Read the model definition and answer for the solid it produces. Units are mm, in the model's axes. A direction names the side the tool comes from. Round coordinates to 2 decimals unless told otherwise and drop trailing zeros. Order: outer loops, then holes, each group sorted by start corner. A loop starts at its lowest first (then second) coordinate and runs counter-clockwise, first axis right, second up.
from build123d import *

# Parameters (mm, degrees)
SKETCH_W        = 200
SKETCH_H        = 90
SKETCH_R        = 1.5625
SKETCH_W_2      = 60
SKETCH_H_2      = 67
PAD_DEPTH       = 5
SKETCH002_W     = 41
SKETCH002_H     = 9.5
POCKET_DEPTH    = 5.001
SKETCH003_R     = 1.5625
POCKET001_DEPTH = 5.001
FILLET_R        = 30
FILLET001_R     = 4
FILLET002_R     = 4
FILLET003_R     = 4


with BuildPart() as part:
    # Sketch → Pad (new body)
    with BuildSketch(Plane.XY):
        with Locations((100, -45)):
            Rectangle(SKETCH_W, SKETCH_H)
        with Locations((185, -30)):
            Circle(SKETCH_R, mode=Mode.SUBTRACT)
        with Locations((185, -10)):
            Circle(SKETCH_R, mode=Mode.SUBTRACT)
        with Locations((175, -20)):
            Circle(SKETCH_R, mode=Mode.SUBTRACT)
        with Locations((175, -40)):
            Circle(SKETCH_R, mode=Mode.SUBTRACT)
        with Locations((25, -40)):
            Circle(SKETCH_R, mode=Mode.SUBTRACT)
        with Locations((25, -20)):
            Circle(SKETCH_R, mode=Mode.SUBTRACT)
        with Locations((15, -30)):
            Circle(SKETCH_R, mode=Mode.SUBTRACT)
        with Locations((15, -10)):
            Circle(SKETCH_R, mode=Mode.SUBTRACT)
        with Locations((70, -38.5)):
            Rectangle(SKETCH_W_2, SKETCH_H_2, mode=Mode.SUBTRACT)
        with BuildLine():
            ThreePointArc((158.0113, -7.9887), (155.0113, -4.9887), (152.0113, -7.9887))
            Line((152.0113, -7.9887), (152.0113, -17.9887))
            ThreePointArc((152.0113, -17.9887), (155.0113, -20.9887), (158.0113, -17.9887))
            Line((158.0113, -7.9887), (158.0113, -17.9887))
        make_face(mode=Mode.SUBTRACT)
        with BuildLine():
            ThreePointArc((151, -31.5), (131.5, -12), (112, -31.5))
            Line((112, -31.5), (112, -41.5))
            ThreePointArc((112, -41.5), (131.5, -61), (151, -41.5))
            Line((151, -31.5), (151, -41.5))
        make_face(mode=Mode.SUBTRACT)
        with BuildLine():
            ThreePointArc((158.0113, -55.0113), (155.0113, -52.0113), (152.0113, -55.0113))
            Line((152.0113, -55.0113), (152.0113, -65.0113))
            ThreePointArc((152.0113, -65.0113), (155.0113, -68.0113), (158.0113, -65.0113))
            Line((158.0113, -55.0113), (158.0113, -65.0113))
        make_face(mode=Mode.SUBTRACT)
        with BuildLine():
            ThreePointArc((110.9887, -55.0113), (107.9887, -52.0113), (104.9887, -55.0113))
            Line((104.9887, -55.0113), (104.9887, -65.0113))
            ThreePointArc((104.9887, -65.0113), (107.9887, -68.0113), (110.9887, -65.0113))
            Line((110.9887, -55.0113), (110.9887, -65.0113))
        make_face(mode=Mode.SUBTRACT)
        with BuildLine():
            ThreePointArc((110.9887, -7.9887), (107.9887, -4.9887), (104.9887, -7.9887))
            Line((104.9887, -7.9887), (104.9887, -17.9887))
            ThreePointArc((104.9887, -17.9887), (107.9887, -20.9887), (110.9887, -17.9887))
            Line((110.9887, -7.9887), (110.9887, -17.9887))
        make_face(mode=Mode.SUBTRACT)
    extrude(amount=PAD_DEPTH)

    # Sketch002 → Pocket (cut, through all)
    with BuildSketch(Plane.XY.offset(5)):
        with Locations((70, -76.75)):
            Rectangle(SKETCH002_W, SKETCH002_H)
    extrude(amount=-POCKET_DEPTH, mode=Mode.SUBTRACT)

    # Sketch003 → Pocket001 (cut, through all)
    with BuildSketch(Plane.XY.offset(5)):
        with Locations((25, -10)):
            Circle(SKETCH003_R)
        with Locations((15, -20)):
            Circle(SKETCH003_R)
        with Locations((15, -40)):
            Circle(SKETCH003_R)
        with Locations((25, -30)):
            Circle(SKETCH003_R)
        with Locations((175, -10)):
            Circle(SKETCH003_R)
        with Locations((185, -20)):
            Circle(SKETCH003_R)
        with Locations((185, -40)):
            Circle(SKETCH003_R)
        with Locations((175, -30)):
            Circle(SKETCH003_R)
    extrude(amount=-POCKET001_DEPTH, mode=Mode.SUBTRACT)

    # Fillet
    fillet_edges = [part.edges().sort_by_distance(p)[0] for p in [
        (200, -90, 2.5),
        (0, -90, 2.5),
    ]]
    fillet(fillet_edges, radius=FILLET_R)

    # Fillet001
    fillet001_edges = [part.edges().sort_by_distance(p)[0] for p in [
        (40, -72, 2.5),
        (49.5, -81.5, 2.5),
        (49.5, -72, 2.5),
        (100, -72, 2.5),
        (90.5, -72, 2.5),
        (90.5, -81.5, 2.5),
    ]]
    fillet(fillet001_edges, radius=FILLET001_R)

    # Fillet002
    fillet002_edges = [part.edges().sort_by_distance(p)[0] for p in [
        (0, 0, 2.5),
        (200, 0, 2.5),
    ]]
    fillet(fillet002_edges, radius=FILLET002_R)

    # Fillet003
    fillet003_edges = [part.edges().sort_by_distance(p)[0] for p in [
        (40, -5, 2.5),
        (100, -5, 2.5),
    ]]
    fillet(fillet003_edges, radius=FILLET003_R)


solid = part.part
Q1. For a pull along X with two mould halves and no side action, classify faces 1 (the face through (158.011, -60, 2)), 2 (the face through (1.141, -1.203, 2.535)) as released by +X, released by -X, zero draft, split by the parting line, or undercut.
Outcome:
face 1: undercut
face 2: released by -X
Q2. Flat-ended cylindrical pins translate along their axes: pin 1 (1.2 mm diameter, centred on y = -76.5, z = 1.5, fed in from +X); pin 2 (1.9 mm diameter, centred on x = 185, y = -30, fed in from +Z); pin 3 (1.5 mm diameter, centred on y = -61.5, z = 3.5, fed in from -X). Find the tip coordinate at first contact, or state that the pin passes through.
Outcome:
pin 1: stops at x = 195.44
pin 2: passes through
pin 3: stops at x = 0.01
Q3. A cutting plane is placed at D-D, the plane x = 156. Give the vertices of the cut face in (y, z), plus the area to 3 significant figures.
Outcome:
outline: (-90, 0) - (-67.84, 0) - (-67.84, 5) - (-90, 5) - close; (-52.18, 0) - (-20.82, 0) - (-20.82, 5) - (-52.18, 5) - close; (-5.16, 0) - (0, 0) - (0, 5) - (-5.16, 5) - close
area: 293 mm2
Q4. A cutting plane is placed at A-A, the plane x = 131.5. Give the vertices of the cut face in (y, z).
Outcome:
outline: (-90, 0) - (-61, 0) - (-61, 5) - (-90, 5) - close; (-12, 0) - (0, 0) - (0, 5) - (-12, 5) - close
Q5. A cutting plane is placed at B-B, the plane y = -36. Give the vertices of the cut face in (x, z), plus the area to 3 significant figures.
Outcome:
outline: (0, 0) - (40, 0) - (40, 5) - (0, 5) - close; (100, 0) - (112, 0) - (112, 5) - (100, 5) - close; (151, 0) - (200, 0) - (200, 5) - (151, 5) - close
area: 505 mm2
Q6. A cutting plane is placed at C-C, the plane z = 2.05. Give the number of separate pieces and of enclosed holes in the cut face, plus the area to 3 significant figures.
Outcome:
separate pieces: 1
enclosed holes: 22
area: 11,200 mm2
Q7. Straight lines are drawn through the part: probe 1 along Y at (x, z) = (60, 3.8); probe 2 along Y at (x, z) = (25, 1.8); probe 3 along Y at (x, z) = (155.5, 4.8). For each, find the intervals that lie inside material, in ascending order.
Outcome:
probe 1: y = -90 to -81.5, -5 to 0
probe 2: y = -89.58 to -41.56, -38.44 to -31.56, -28.44 to -21.56, -18.44 to -11.56, -8.44 to 0
probe 3: y = -90 to -67.97, -52.05 to -20.95, -5.03 to 0
Q8. For faces 3 (the face through (104.989, -13, 2)), 4 (the face through (8.555, -80.979, 2.535)), determine the directions among +Z, -Z, +X, -X, +Y, -Y from which every point of the face is accessible in a straight line to the end or side of a thin tool.
Outcome:
face 3: +Z, -Z
face 4: +Z, -Z, -X, -Y
